Print and shaded views of the part. All mm, measured from the part's lowest x, y and z. Round coordinates to 2 decimals unless told otherwise and drop trailing zeros. Write each loop counter-clockwise with the first axis right and the second up, starting at its lowest first coordinate (ties: lowest second). Pieces come first, ordered by that corner, then holes. Notation, with made-up numbers: (1.25, 22.5) - (57.25, 22.5) arc R16 cw to (57.25, 38.5) - close; hole circle Ø11 at (7, 76.5). An arc over 180 degrees is marked (long way). Put each result on its own line as item: value. Start each with the question number.
Item 1: Cut at B-B (x = 88). Give the cut face in (y, z), and give its area (3 significant figures).
Item 2: Cut at C-C (x = 5). Give the cut face in (y, z), and give its area (3 significant figures).
Item 3: Cut at A-A (z = 24.5). Give the cut face in (x, y), and give its area (3 significant figures).
Item 4: Cut at D-D (z = 75). Give the cut face in (x, y).
Item 5: Drill centre lines: line 1 (X direction, y = 5.2, z = 75); line 2 (Z direction, x = 11, y = 4.1); line 3 (X direction, y = 5.4, z = 66). Where is each one in solid material? Low to high. Write a range as from..to.
Item 6: Pin check, flat tip, straight feed: pin 1 Ø4 at (x, z) = (95.5, 76.5) entering from +Y. Stop position of the tip, or through.
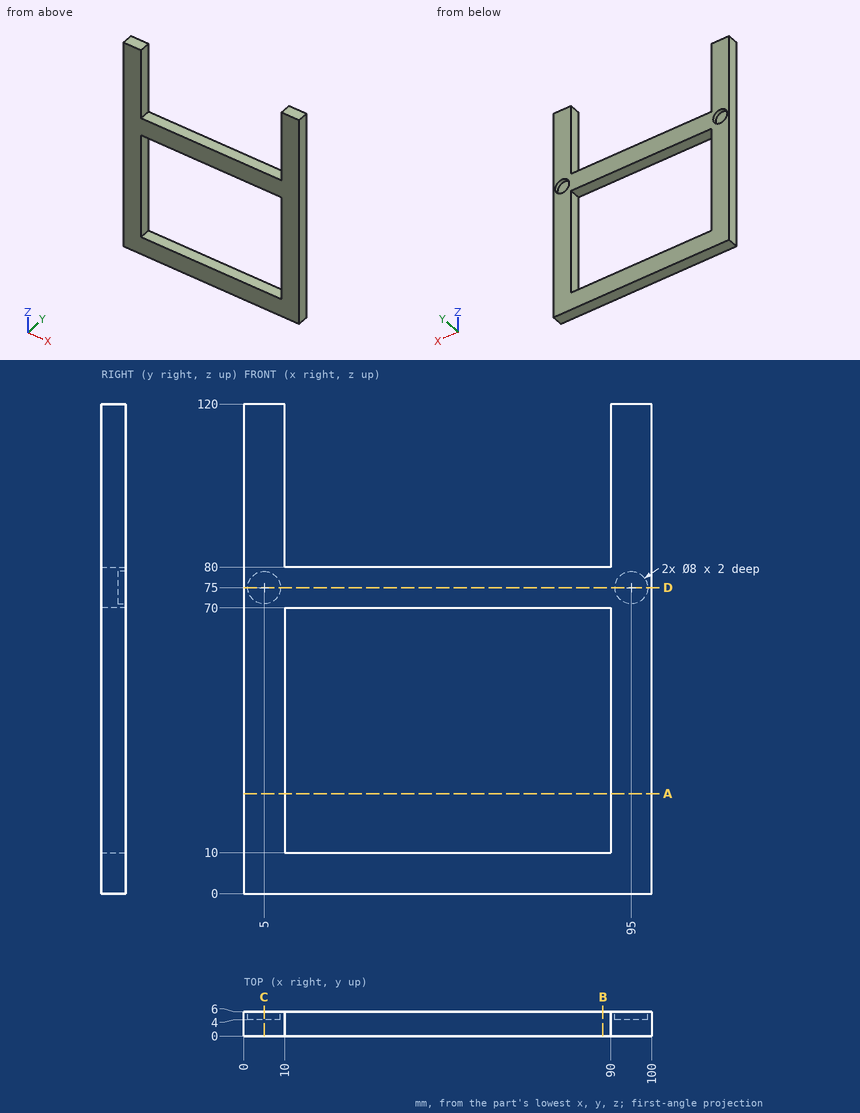
Output values:
1. outline: (0, 0) - (6, 0) - (6, 10) - (0, 10) - close; (0, 70) - (6, 70) - (6, 80) - (0, 80) - close
1. area: 120 mm2
2. outline: (0, 0) - (6, 0) - (6, 71) - (4, 71) - (4, 79) - (6, 79) - (6, 120) - (0, 120) - close
2. area: 704 mm2
3. outline: (0, 0) - (10, 0) - (10, 6) - (0, 6) - close; (90, 0) - (100, 0) - (100, 6) - (90, 6) - close
3. area: 120 mm2
4. outline: (0, 0) - (100, 0) - (100, 6) - (99, 6) - (99, 4) - (91, 4) - (91, 6) - (9, 6) - (9, 4) - (1, 4) - (1, 6) - (0, 6) - close
5. line 1: 0..1, 9..91, 99..100
5. line 2: 0..10, 70..80
5. line 3: 0..10, 90..100
6. pin 1: y = 4
